Print and shaded views of the part. All mm, measured from the part's lowest x, y and z. A direction names the side the tool comes from. Give positions to 0.01 mm unless a question says otherwise; leave off trailing zeros. Loops run counter-clockwise (first coordinate to the right, second up) from the corner with the lowest first, then second, coordinate; pieces in that order, holes last. Notation, with made-up numbers: (82, 25) - (103, 25) arc R14 ccw to (103, 31) - close; hole circle Ø1 at (-21.5, 27). An arc over 180 degrees is marked (long way). Return JSON: item names as keys, results as strings.
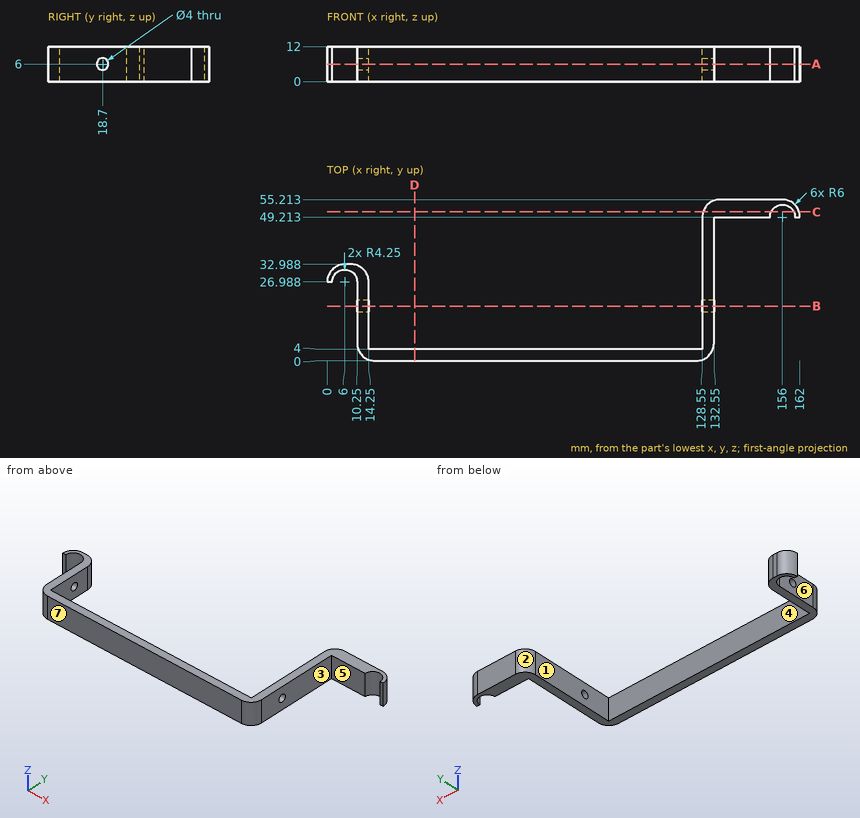
1. Pull direction X, two halves, no side cores. Call the marked faces 1, 2, 3 and 4: +X half, -X half, draft (parallel to the pull), parting line (faces both ways), or undercut.
Values follow:
{"face 1": "undercut", "face 2": "-X half", "face 3": "+X half", "face 4": "undercut"}
2. Cut at D-D, the plane x = 30. Write the cut outline in (y, z), plus the area to 3 significant figures.
Values follow:
{"outline": "(0, 0) - (4, 0) - (4, 12) - (0, 12) - close", "area": "48.0 mm²"}
3. Cut at A-A, the plane z = 6. Write the cut outline in (x, y).
Values follow:
{"outline": "(0, 26.99) - (1.75, 26.99) arc R4.25 cw to (10.25, 26.99) - (10.25, 20.7) - (14.25, 20.7) - (14.25, 26.99) arc R6 ccw to (8.25, 32.99) - (6, 32.99) arc R6 ccw to start; (10.25, 6) arc R6 ccw to (16.25, 0) - (126.55, 0) arc R6 ccw to (132.55, 6) - (132.55, 16.7) - (128.55, 16.7) - (128.55, 4) - (14.25, 4) - (14.25, 16.7) - (10.25, 16.7) - close; (128.55, 20.7) - (132.55, 20.7) - (132.55, 49.21) - (151.75, 49.21) arc R4.25 cw to (160.25, 49.21) - (162, 49.21) arc R6 ccw to (156, 55.21) - (134.55, 55.21) arc R6 ccw to (128.55, 49.21) - close"}
4. Which spindle directions (+Z, -Z, +X, -X, +Y, -Y) get a long thin tool onto all of the face, cutting with end or side? Do the marked faces 5, 6 and 7. Say none if no direction does.
Values follow:
{"face 5": "+Z, -Z, +X, -Y", "face 6": "+Z, -Z, -X, -Y", "face 7": "+Z, -Z, +X, -X, -Y"}
5. Cut at B-B, the plane y = 18.7. Write the cut outline in (x, z).
Values follow:
{"outline": "(10.25, 0) - (14.25, 0) - (14.25, 4) - (10.25, 4) - close; (10.25, 8) - (14.25, 8) - (14.25, 12) - (10.25, 12) - close; (128.55, 0) - (132.55, 0) - (132.55, 4) - (128.55, 4) - close; (128.55, 8) - (132.55, 8) - (132.55, 12) - (128.55, 12) - close"}
6. Drill centre lines: probe 1 along X at (y, z) = (25.5, 2); probe 2 along Z at (x, y) = (130.55, 18.7); probe 3 along Y at (x, z) = (122, 7). Where is each one in solid material? Low to high.
Values follow:
{"probe 1": "x = 10.25 to 14.25, 128.55 to 132.55", "probe 2": "z = 0 to 4, 8 to 12", "probe 3": "y = 0 to 4"}
7. Drop flat-ended pins along their axis: P1, Ø1.1, axis at x = 7, z = 7.5, coming from the +Y side; P2, Ø1.5, axis at x = 127.5, z = 8.5, coming from the +Y side; P3, Ø4.5, axis at y = 18.7, z = 6, coming from the -X side. Give the stop position or say it passes through.
Values follow:
{"P1": "stops at y = 32.99", "P2": "stops at y = 4", "P3": "stops at x = 10.25"}
8. Cut at C-C, the plane y = 51. Write the cut outline in (x, z) (1 decimal), plus the area to 3 significant figures.
Values follow:
{"outline": "(128.8, 0) - (152.1, 0) - (152.1, 12) - (128.8, 12) - close; (159.9, 0) - (161.7, 0) - (161.7, 12) - (159.9, 12) - close", "area": "302 mm²"}
